Can you work these out from the drawing? Everything is in mm from the part's minimum corner. A direction names the side the tool comes from. Round coordinates to 2 decimals unless told otherwise and drop trailing zeros. Order: outer loops, then holes, each group sorted by start corner. A loop starts at its lowest first (then second) coordinate and runs counter-clockwise, first axis right, second up. Notation, with made-up numbers: M -34,14 L 9,14 A15 ccw 9,22 Z; hole C 42.5,21 d1. An arc over 180 degrees is marked long. Write item = value, one per line. Start each with the question number.
Item 1: I'm going to push flat-ended pins straight in: P1, Ø6, axis at x = 10.5, y = 14, coming from the +Z side; P2, Ø4.5, axis at x = 24, z = 6.5, coming from the -Y side; P3, Ø10, axis at y = 18, z = 10.5, coming from the +X side; P4, Ø3, axis at x = 28, y = 39.5, coming from the +Z side. Where does each tip first touch, or does it pass through?
Item 2: I want a section at B-B, the plane z = 4.5. List the corners of the cut face in (x, y) for me, plus the area to 3 significant figures.
Item 3: Please list where these lines run through material, in increasing order: L1, parallel to Z at x = 3.25, y = 5; L2, parallel to Z at x = 48.6, y = 43.75; L3, parallel to Y at x = 50, z = 8.
Item 4: I want a section at A-A, the plane z = 16.1. List the corners of the cut face in (x, y) for me.
Item 5: For the marked faces 1, 2 and 3, which set-ups out of +Z, -Z, +X, -X, +Y, -Y let a thin tool reach every point of the face, with its end or its side?
Item 6: I want a section at C-C, the plane x = 48.6. List the corners of the cut face in (y, z) for me.
Item 7: I want a section at D-D, the plane y = 30. List the corners of the cut face in (x, z) for me, plus the area to 3 significant figures.
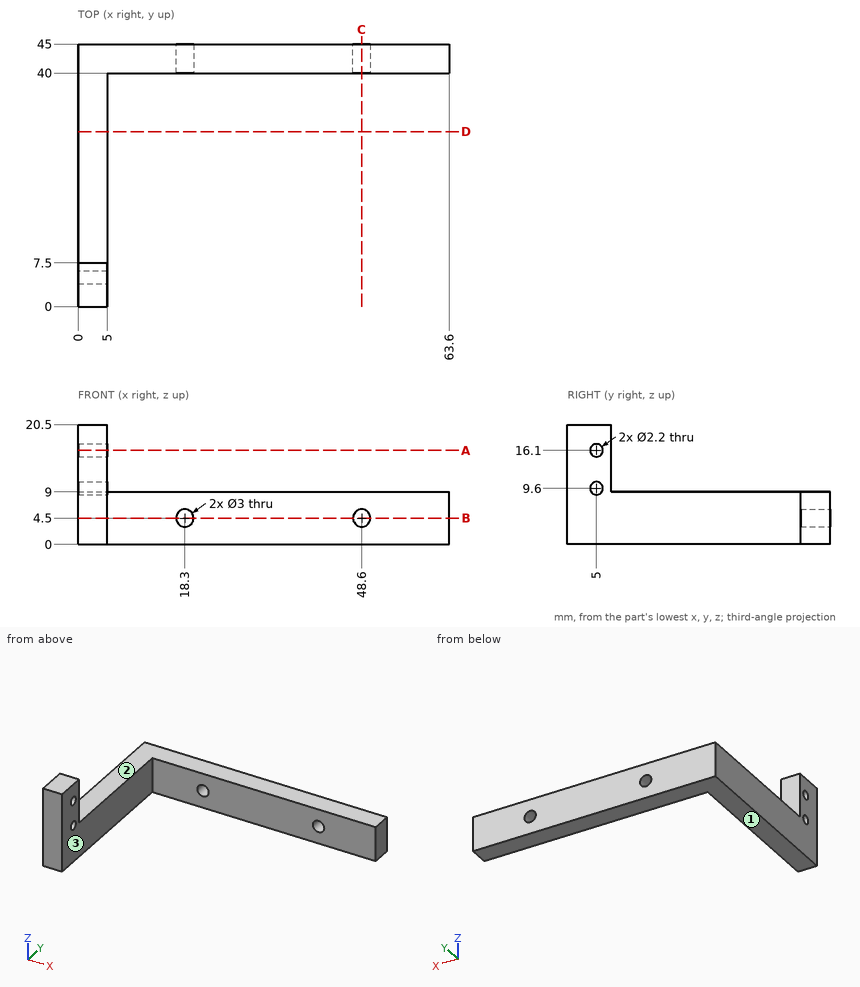
Filled in:
q1.P1 = through
q1.P2 = 40
q1.P3 = 5
q1.P4 = 9
q2.outline = M 0,0 L 5,0 L 5,40 L 16.8,40 L 16.8,45 L 0,45 Z; M 19.8,40 L 47.1,40 L 47.1,45 L 19.8,45 Z; M 50.1,40 L 63.6,40 L 63.6,45 L 50.1,45 Z
q2.area = 488 mm^2
q3.L1 = 0 to 8.5, 10.7 to 15, 17.2 to 20.5
q3.L2 = 0 to 3, 6 to 9
q3.L3 = 40 to 45
q4.outline = M 0,0 L 5,0 L 5,3.9 L 0,3.9 Z; M 0,6.1 L 5,6.1 L 5,7.5 L 0,7.5 Z
q5.face_1 = -Z, +X, -X, +Y, -Y
q5.face_2 = +Z, +X, -X, +Y
q5.face_3 = +Z, -Z, +X, -Y
q6.outline = M 40,0 L 45,0 L 45,3 L 40,3 Z; M 40,6 L 45,6 L 45,9 L 40,9 Z
q7.outline = M 0,0 L 5,0 L 5,9 L 0,9 Z
q7.area = 45.0 mm^2
